from build123d import *

# Parameters (mm, degrees)
SKETCH028_W        = 71
SKETCH028_H        = 81
PAD014_DEPTH       = 5
SKETCH034_W        = 68
SKETCH034_H        = 1.5
PAD017_DEPTH       = 2
SKETCH035_W        = 64.6
SKETCH035_H        = 77.6
PAD018_DEPTH       = 2
SKETCH036_W        = 50
SKETCH036_H        = 72
POCKET028_DEPTH    = 4
SKETCH039_W        = 7.3
SKETCH039_H        = 10
PAD020_DEPTH       = 9
SKETCH040_W        = 5
SKETCH040_H        = 3.5
PAD021_DEPTH       = 9
CHAMFER006_SIZE    = 4.9
SKETCH041_R        = 2.5
POCKET031_DEPTH    = 10
SKETCH047_R        = 2.5
POCKET043_DEPTH    = 10
SKETCH051_R        = 4.5
POCKET044_DEPTH    = 3
POCKET044_FACE29_W = 64.6
POCKET044_FACE29_H = 2
POCKET045_DEPTH    = 2
POCKET045_FACE16_W = 50
POCKET045_FACE16_H = 4
PAD035_DEPTH       = 2
POCKET046_DEPTH    = 2
CHAMFER012_SIZE    = 3
CHAMFER018_SIZE    = 2
SKETCH063_W        = 50
SKETCH063_H        = 72
PAD040_DEPTH       = 2
PAD040_FACE37_W    = 0.5
PAD040_FACE37_H    = 50
POCKET056_DEPTH    = 0.5
PAD042_DEPTH       = 0.5
PAD043_DEPTH       = 0.5
POCKET064_DEPTH    = 1
CHAMFER022_SIZE    = 0.999
FILLET006_R        = 3


with BuildPart() as part:
    # Sketch028 → Pad014 (new body)
    with BuildSketch(Plane.XY):
        with Locations((-0.121221, -9.466726)):
            Rectangle(SKETCH028_W, SKETCH028_H)
    extrude(amount=-PAD014_DEPTH)

    # Sketch034 (on Face1 of Pad014) → Pad017 (join)
    with BuildSketch(Plane(origin=(0, 31.033274, 0), x_dir=(-1, 0, 0), z_dir=(0, 1, 0))):
        with Locations((0.121221, -0.75)):
            Rectangle(SKETCH034_W, SKETCH034_H)
    extrude(amount=PAD017_DEPTH)

    # Sketch035 (on Face10 of Pad017) → Pad018 (join)
    with BuildSketch(Plane.XY):
        with Locations((-0.121221, -5.766726)):
            Rectangle(SKETCH035_W, SKETCH035_H)
    extrude(amount=PAD018_DEPTH)

    # Sketch036 (on Face13 of Pad018) → Pocket028 (cut)
    with BuildSketch(Plane.XY.offset(2)):
        with Locations((-0.121221, -6.466726)):
            Rectangle(SKETCH036_W, SKETCH036_H)
    extrude(amount=-POCKET028_DEPTH, mode=Mode.SUBTRACT)

    # Sketch039 (on Face14 of Pocket028) → Pad020 (join)
    with BuildSketch(Plane.XY.offset(2)):
        with Locations((28.528779, 28.033274)):
            Rectangle(SKETCH039_W, SKETCH039_H)
        with Locations((-28.771221, 28.033274)):
            Rectangle(SKETCH039_W, SKETCH039_H)
    extrude(amount=PAD020_DEPTH)

    # Sketch040 (on Face1 of Pad020) → Pad021 (join)
    with BuildSketch(Plane.XY.offset(2)):
        with Locations((-22.621221, 31.283274)):
            Rectangle(SKETCH040_W, SKETCH040_H)
        with Locations((22.378779, 31.283274)):
            Rectangle(SKETCH040_W, SKETCH040_H)
    extrude(amount=PAD021_DEPTH)

    # Chamfer006
    chamfer006_edges = [part.edges().sort_by_distance(p)[0] for p in [
        (-20.121221, 31.283274, 11),
        (19.878779, 31.283274, 11),
    ]]
    chamfer(chamfer006_edges, length=CHAMFER006_SIZE)

    # Sketch041 (on Face12 of Chamfer006) → Pocket031 (cut)
    with BuildSketch(Plane(origin=(0, 33.033274, 0), x_dir=(-1, 0, 0), z_dir=(0, 1, 0))):
        with Locations((-28.378779, 6)):
            Circle(SKETCH041_R)
        with Locations((28.621221, 6)):
            Circle(SKETCH041_R)
    extrude(amount=-POCKET031_DEPTH, mode=Mode.SUBTRACT)

    # Sketch047 (on Face30 of Pocket031) → Pocket043 (cut)
    with BuildSketch(Plane(origin=(0, 0, -5), x_dir=(1, 0, 0), z_dir=(0, 0, -1))):
        with Locations((-28.621221, 30.966726)):
            Circle(SKETCH047_R)
        with Locations((28.378779, 30.966726)):
            Circle(SKETCH047_R)
    extrude(amount=-POCKET043_DEPTH, mode=Mode.SUBTRACT)

    # Sketch051 (on Face32 of Pocket043) → Pocket044 (cut)
    with BuildSketch(Plane(origin=(0, 0, -5), x_dir=(1, 0, 0), z_dir=(0, 0, -1))):
        with Locations((-28.621221, 30.966726)):
            Circle(SKETCH051_R)
        with Locations((28.378779, 30.966726)):
            Circle(SKETCH051_R)
    extrude(amount=-POCKET044_DEPTH, mode=Mode.SUBTRACT)

    # Pocket044 Face29 → Pocket045 (cut)
    with BuildSketch(Plane(origin=(-0.121221, -44.566726, 1), x_dir=(-1, 0, 0), z_dir=(0, -1, 0))):
        Rectangle(POCKET044_FACE29_W, POCKET044_FACE29_H)
    extrude(amount=-POCKET045_DEPTH, mode=Mode.SUBTRACT)

    # Pocket045 Face16 → Pad035 (add)
    with BuildSketch(Plane(origin=(-0.121221, -42.466726, 0), x_dir=(1, 0, 0), z_dir=(0, 1, 0))):
        Rectangle(POCKET045_FACE16_W, POCKET045_FACE16_H)
    extrude(amount=PAD035_DEPTH)

    # Pad035 Face1 → Pocket046 (cut)
    with BuildSketch(Plane(origin=(-0.121221, 29.533274, 1.353834), x_dir=(-1, 0, 0), z_dir=(0, -1, 0))):
        Polygon((-25, -9.646166), (-24.9, -9.646166), (-20, -4.746166), (-20, -0.646166), (20, -0.646166), (20, -4.746166), (24.9, -9.646166), (25, -9.646166), (25, 3.353834), (-25, 3.353834), align=None)
    extrude(amount=-POCKET046_DEPTH, mode=Mode.SUBTRACT)

    # Chamfer012
    chamfer012_edges = [part.edges().sort_by_distance(p)[0] for p in [
        (-0.121221, -49.966726, -5),
    ]]
    chamfer(chamfer012_edges, length=CHAMFER012_SIZE)

    # Chamfer018
    chamfer018_edges = [part.edges().sort_by_distance(p)[0] for p in [
        (-28.771221, 23.033274, 11),
        (28.528779, 23.033274, 11),
    ]]
    chamfer(chamfer018_edges, length=CHAMFER018_SIZE)

    # Sketch063 (on Face10 of Chamfer018) → Pad040 (join)
    with BuildSketch(Plane.XY.offset(-2)):
        with Locations((-0.121221, -4.466726)):
            Rectangle(SKETCH063_W, SKETCH063_H)
    extrude(amount=PAD040_DEPTH)

    # Pad040 Face37 → Pocket056 (cut)
    with BuildSketch(Plane(origin=(-0.121221, 31.283274, -2), x_dir=(0, -1, 0), z_dir=(0, 0, -1))):
        Rectangle(PAD040_FACE37_W, PAD040_FACE37_H)
    extrude(amount=-POCKET056_DEPTH, mode=Mode.SUBTRACT)

    # Pocket056 Face9 → Pad042 (add)
    with BuildSketch(Plane(origin=(-32.421221, 7.336396, 2.99136), x_dir=(0, 1, 0), z_dir=(-1, 0, 0))):
        Polygon((17.696878, -8.00864), (25.696878, -8.00864), (25.696878, 2.99136), (-49.903122, 2.99136), (-49.903122, 0.99136), (15.696878, 0.99136), (15.696878, -6.00864), align=None)
    extrude(amount=PAD042_DEPTH)

    # Pad042 Face19 → Pad043 (add)
    with BuildSketch(Plane(origin=(32.178779, 7.336396, 2.99136), x_dir=(0, -1, 0), z_dir=(1, 0, 0))):
        Polygon((-15.696878, -6.00864), (-15.696878, 0.99136), (49.903122, 0.99136), (49.903122, 2.99136), (-25.696878, 2.99136), (-25.696878, -8.00864), (-17.696878, -8.00864), align=None)
    extrude(amount=PAD043_DEPTH)

    # Sketch066 (on Face22 of Pad043) → Pocket064 (cut)
    with BuildSketch(Plane(origin=(0, 0, -5), x_dir=(1, 0, 0), z_dir=(0, 0, -1))):
        with BuildLine():
            ThreePointArc((-5.121221, 34), (-0.121221, 28.999784), (4.878779, 34))
            Line((-5.121221, 34), (4.878779, 34))
        make_face()
    extrude(amount=-POCKET064_DEPTH, mode=Mode.SUBTRACT)

    # Chamfer022
    chamfer022_edges = [part.edges().sort_by_distance(p)[0] for p in [
        (-0.121221, -28.999784, -5),
    ]]
    chamfer(chamfer022_edges, length=CHAMFER022_SIZE)

    # Fillet006
    fillet006_edges = [part.edges().sort_by_distance(p)[0] for p in [
        (-35.621221, -7.966726, -5),
        (35.378779, -7.966726, -5),
    ]]
    fillet(fillet006_edges, radius=FILLET006_R)


with BuildPart() as part_1:
    # Body004 placement: moved
    add(part.part.moved(Location((0.1, -10.49, -34))))


solid = part_1.part
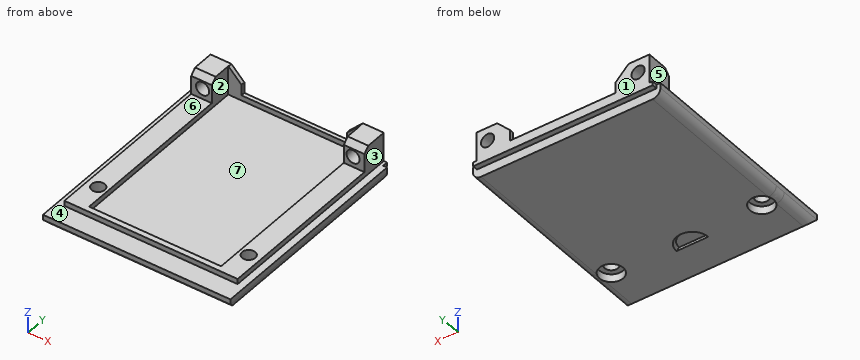
The model under review builds one solid part; all positions refer to its coordinate system, in mm. Face numbers are marked on the shaded views. A direction names the side the tool comes from. Coordinates: 2 decimals unless noted, no trailing zeros. Loops run counter-clockwise (first coordinate to the right, second up) from the corner with the lowest first, then second, coordinate; pieces in that order, holes last. Notation, with made-up numbers: (-38, -18) -> (14, -18) arc R22 cw to (14, 6) -> close; hole circle Ø9 at (-23.75, 61.5). An arc over 180 degrees is marked (long way). Use a Markdown table: item, result. Add a question column.
1. Clearance check with flat-ended pins moving along their axes: pin 1 Ø1 at (x, y) = (-26.5, -39.5) entering from -Z; pin 2 Ø6 at (x, y) = (14, -50) entering from +Z; pin 3 Ø19.5 at (x, y) = (1, -8) entering from +Z; pin 4 Ø1.5 at (y, z) = (-47.5, -30.5) entering from +X. State where each tip first meets the part, or that it passes through.
2. Add section A-A on z = -27. Write out the cut boundary in (x, y), plus the area to 3 significant figures.
3. Draft analysis for pull direction Y (two halves, no side actions). For the marked faces 1, 2 and 3, state which applies: pulls with the +Y half, pulls with the -Y half, needs draft (parallel to the pull), parting line crosses it, or undercut.
4. Add section B-B on y = -36. Write out the cut boundary in (x, z).
5. To check wall thickness, follow line 1 (Y direction, x = 1.5, z = -33.5); line 2 (X direction, y = 16, z = -24.75); line 3 (Z direction, x = -11, y = -55). State the ranges of each line that lie inside material, in increasing order.
6. Machinability: for the marked faces 4, 5, 6 and 7, which of the approach directions +Z, -Z, +X, -X, +Y, -Y give a long, thin tool a straight path to every point of the face, cutting with its end or side? Answer none if there is none.
Returned:
| question | item | result |
|---|---|---|
| 1 | pin 1 | stops at z = -36 |
| 1 | pin 2 | stops at z = -32 |
| 1 | pin 3 | stops at z = -34 |
| 1 | pin 4 | passes through |
| 2 | outline | (-32.82, 12.54) -> (-30.81, 12.54) -> (-30.81, 22.54) -> (-32.82, 22.54) -> close; (-26.23, 12.54) -> (-25.02, 12.54) -> (-25.02, 21.04) -> (-20.92, 21.04) -> (-20.92, 22.54) -> (-26.23, 22.54) -> close; (20.88, 21.04) -> (24.98, 21.04) -> (24.98, 12.54) -> (26.19, 12.54) -> (26.19, 22.54) -> (20.88, 22.54) -> close; (30.77, 12.54) -> (32.78, 12.54) -> (32.78, 22.54) -> (30.77, 22.54) -> close |
| 2 | area | 76.6 mm² |
| 3 | face 1 | pulls with the +Y half |
| 3 | face 2 | undercut |
| 3 | face 3 | needs draft |
| 4 | outline | (-35.52, -36) arc R3 ccw to (-32.52, -39) -> (32.48, -39) arc R3 ccw to (35.48, -36) -> (35.48, -34) -> (32.78, -34) -> (32.78, -32) -> (24.98, -32) -> (24.98, -34) -> (-25.02, -34) -> (-25.02, -32) -> (-32.82, -32) -> (-32.82, -34) -> (-35.52, -34) -> close |
| 5 | line 1 | y = -53.06 to -50.96, 21.04 to 22.54 |
| 5 | line 2 | x = -32.82 to -25.02, 24.98 to 32.78 |
| 5 | line 3 | z = -39 to -34 |
| 6 | face 4 | +Z, -Y |
| 6 | face 5 | +Z, -X, +Y, -Y |
| 6 | face 6 | +Z, +X, -X, -Y |
| 6 | face 7 | +Z |
